```python
from build123d import *

# Parameters (mm, degrees)
SKETCH1_R           = 0.1
BOSS_EXTRUDE1_DEPTH = 0.18
FILLET2_R           = 0.5


with BuildPart() as part:
    # Sketch1 → Boss-Extrude1 (new body)
    with BuildSketch(Plane(origin=(0, 0, 0), x_dir=(1, 0, 0), z_dir=(0, 1, 0))):
        with BuildLine():
            Line((-0.3, -3.969693846), (-0.3, -1.469693846))
            ThreePointArc((-0.3, -1.469693846), (-1.5, 0), (-0.3, 1.469693846))
            Line((-0.3, 1.469693846), (-0.3, 15.530306154))
            Line((-0.3, 15.530306154), (0.3, 15.530306154))
            Line((0.3, 15.530306154), (0.3, 1.469693846))
            ThreePointArc((0.3, 1.469693846), (1.5, 0), (0.3, -1.469693846))
            Line((0.3, -1.469693846), (0.3, -3.969693846))
            Line((0.3, -3.969693846), (-0.3, -3.969693846))
        make_face()
        with Locations(Location((0, 0, 0), (0, 0, 270))):
            Circle(SKETCH1_R, mode=Mode.SUBTRACT)
    extrude(amount=BOSS_EXTRUDE1_DEPTH)

    # Fillet2
    # the kernel refuses this fillet: 0.5 mm, written as the material it takes off along each edge
    with BuildSketch(Plane(origin=(-0.3, -1.25, -15.530306154), x_dir=(0, 0, 1), z_dir=(0, 1, 0)), Plane(origin=(0.3, -1.25, -15.530306154), x_dir=(-1, 0, 0), z_dir=(0, 1, 0)), Plane(origin=(-0.3, -1.25, 3.969693846), x_dir=(1, 0, 0), z_dir=(0, 1, 0)), Plane(origin=(0.3, -1.25, 3.969693846), x_dir=(0, 0, -1), z_dir=(0, 1, 0))) as fillet2_piece_1:
        with BuildLine():
            CenterArc((FILLET2_R, FILLET2_R), FILLET2_R, 180, 90)
            Line((0, FILLET2_R), (0, 0))
            Line((0, 0), (FILLET2_R, 0))
        make_face()
    extrude(amount=2.68, mode=Mode.SUBTRACT)


solid = part.part
```
CAD build for the part. Positions are in the model's coordinates, mm. Coordinates: 2 decimals unless noted, no trailing zeros. Order: outer loops, then holes, each group sorted by start corner. A loop starts at its lowest first (then second) coordinate and runs counter-clockwise, first axis right, second up. Notation, with made-up numbers: (21, 41) - (33, 41) arc R9 ccw to (33, 55) - close; hole circle Ø8 at (68.5, -9.5). An arc over 180 degrees is marked (long way). Answer in a Markdown table with one row per item.
1. Slice it at C-C, the plane z = 2.5. List the corners of the cut face in (x, y), then the cut area to 3 significant figures.
Answer:
| item | result |
|---|---|
| outline | (-0.3, 0) - (0.3, 0) - (0.3, 0.18) - (-0.3, 0.18) - close |
| area | 0.108 mm² |
2. Drill centre lines: L1, parallel to X at y = 0.05, z = -13.5; L2, parallel to Z at x = 0.2, y = 0.1; L3, parallel to Z at x = 1.3, y = 0.1. Where is each one in solid material? Low to high. Write a range as from..to.
Answer:
| item | result |
|---|---|
| L1 | -0.3..0.3 |
| L2 | -15.33..3.77 |
| L3 | -0.75..0.75 |
3. Slice it at A-A, the plane y = 0.1. List the corners of the cut face in (x, z).
Answer:
| item | result |
|---|---|
| outline | (-0.3, -15.03) arc R0.5 ccw to (0, -15.49) arc R0.5 ccw to (0.3, -15.03) - (0.3, -1.47) arc R1.5 ccw to (0.3, 1.47) - (0.3, 3.47) arc R0.5 ccw to (0, 3.93) arc R0.5 ccw to (-0.3, 3.47) - (-0.3, 1.47) arc R1.5 ccw to (-0.3, -1.47) - close; hole circle Ø0.2 at (0, 0) |
4. Slice it at B-B, the plane x = 1.2. List the corners of the cut face in (y, z).
Answer:
| item | result |
|---|---|
| outline | (0, -0.9) - (0.18, -0.9) - (0.18, 0.9) - (0, 0.9) - close |
